Can you work these out from the model? Positions are in its coordinate system, mm. A direction names the side the tool comes from. Give positions to 0.01 mm unless a question says otherwise; leave off trailing zeros. Order: outer loops, then holes, each group sorted by start corner. A loop starts at its lowest first (then second) coordinate and runs counter-clockwise, first axis right, second up. Notation, with made-up numbers: (67.5, 43.25) - (99.5, 43.25) arc R16 ccw to (99.5, 65.25) - close; hole circle Ø4 at (40, 68.25). An arc over 180 degrees is marked (long way). Answer as a JSON object with one key per item and string values.
```python
from build123d import *

# Parameters (mm, degrees)
F0_W           = 46.776227
F0_H           = 38.1
F1_DEPTH       = 25.4
F2_R           = 7.62
F3_T           = -2.54
F5_D           = 6.35
F5_CSINK_D     = 12.7
F5_CSINK_ANGLE = 100


with BuildPart() as f1:
    # F0 (on Top) → F1 (new body)
    with BuildSketch(Plane.XY):
        with Locations((-0.622407, 0.518654)):
            Rectangle(F0_W, F0_H)
    extrude(amount=F1_DEPTH)

    # F2
    f2_edges = [f1.edges().sort_by_distance(p)[0] for p in [
        (-0.622407, -18.531346, 25.4),
    ]]
    fillet(f2_edges, radius=F2_R)

    # F3
    f3_openings = [f1.faces().sort_by_distance(p)[0] for p in [
        (-0.622407, 0.518654, 0),
    ]]
    offset(amount=F3_T, openings=f3_openings)

    # F5 (through all)
    with Locations(Plane.XY.offset(25.4)):
        with Locations((-12.7, 0), (12.7, 0)):
            CounterSinkHole(F5_D / 2, F5_CSINK_D / 2, counter_sink_angle=F5_CSINK_ANGLE)


solid = f1.part
```
Q1. If we section it at A-A, the plane z = 7.5: Please give me the cut outline in (x, y).
Recorded:
{"outline": "(-24.01, -18.53) - (22.77, -18.53) - (22.77, 19.57) - (-24.01, 19.57) - close; hole (-21.47, -15.99) - (20.23, -15.99) - (20.23, 17.03) - (-21.47, 17.03) - close"}
Q2. We'd pull the mould along Y, two halves only. Please class faces 3 (the face through (-21.471, 0, 11)), 4 (the face through (-5.9, -16.3, 0)), 5 (the face through (-1, -18.531, 9)): released by +Y, released by -Y, zero draft, split by the parting line, or undercut.
Recorded:
{"face 3": "undercut", "face 4": "zero draft", "face 5": "released by -Y"}
Q3. I need wall thicknesses on L1, parallel to Y at x = 15.5, z = 8.5; L2, parallel to X at y = -2, z = 22.75; L3, parallel to Y at x = 2, z = 21.75. Which ranges of each line are inside material? Lowest first, please.
Recorded:
{"L1": "y = -18.53 to -15.99, 17.03 to 19.57", "L2": "x = -24.01 to -21.47, 20.23 to 22.77", "L3": "y = -17.42 to -14.08, 17.03 to 19.57"}
Q4. I'm going to push a flat-ended pin straight in: pin 1 Ø2 at (x, y) = (-10.5, -14.5) entering from -Z. Where does the tip first touch, or does it pass through?
Recorded:
{"pin 1": "stops at z = 19.96"}
Q5. If we section it at D-D, the plane x = 12.7: Please give me the cut outline in (y, z).
Recorded:
{"outline": "(-18.53, 0) - (-15.99, 0) - (-15.99, 17.78) arc R5.08 cw to (-10.91, 22.86) - (-3.32, 22.86) - (-6.35, 25.4) - (-10.91, 25.4) arc R7.62 ccw to (-18.53, 17.78) - close; (3.32, 22.86) - (17.03, 22.86) - (17.03, 0) - (19.57, 0) - (19.57, 25.4) - (6.35, 25.4) - close"}
Q6. If we section it at C-C, the plane y = 10: Please give me the cut outline in (x, z), then the cut area to 3 significant figures.
Recorded:
{"outline": "(-24.01, 0) - (-21.47, 0) - (-21.47, 22.86) - (20.23, 22.86) - (20.23, 0) - (22.77, 0) - (22.77, 25.4) - (-24.01, 25.4) - close", "area": "235 mm^2"}
Q7. If we section it at B-B, the plane x = -2.5: Please give me the cut outline in (y, z), then the cut area to 3 significant figures.
Recorded:
{"outline": "(-18.53, 0) - (-15.99, 0) - (-15.99, 17.78) arc R5.08 cw to (-10.91, 22.86) - (17.03, 22.86) - (17.03, 0) - (19.57, 0) - (19.57, 25.4) - (-10.91, 25.4) arc R7.62 ccw to (-18.53, 17.78) - close", "area": "206 mm^2"}
Q8. Which directions (+Z, -Z, +X, -X, +Y, -Y) give clear straight access to the entire face, cutting with the end or side of a thin tool? Please do faces 1 (the face through (20.226, 0, 11)), 2 (the face through (-24.011, 0, 13)).
Recorded:
{"face 1": "-Z", "face 2": "+Z, -Z, -X, +Y, -Y"}
